Source: CAD feature listing. Evaluate the final solid. Frame: model axes, mm. A direction names the side the tool comes from. Coordinates: 2 decimals unless noted, no trailing zeros. Answer as a JSON object with one key per item and string values. Group by question number.
from build123d import *

# Parameters (mm, degrees)
F1_DEPTH = 7.874
F2_R     = 1.533026
F3_R     = 1.594347
F4_R     = 0.61321


with BuildPart() as f1:
    # F0 (on Front) → F1 (new body)
    with BuildSketch(Plane.XZ):
        Polygon((-7.47635, 9.42706), (-7.47635, 4.603866), (-8.243676, 4.603866), (-8.243676, 9.372251), (-24.138292, 9.372251), (-24.138292, 0), (0, 0), (0, 9.42706), align=None)
    extrude(amount=F1_DEPTH)

    # F2
    f2_edges = [f1.edges().sort_by_distance(p)[0] for p in [
        (-8.243676, -3.937, 9.372251),
    ]]
    fillet(f2_edges, radius=F2_R)

    # F3
    f3_edges = [f1.edges().sort_by_distance(p)[0] for p in [
        (-24.138292, -3.937, 9.372251),
        (-7.47635, -3.937, 9.42706),
    ]]
    fillet(f3_edges, radius=F3_R)

    # F4
    f4_edges = [f1.edges().sort_by_distance(p)[0] for p in [
        (-8.243676, -3.937, 4.603866),
    ]]
    fillet(f4_edges, radius=F4_R)

    # F5: F1 across face


with BuildPart() as f1_1:
    add(f1.part)
    add(f1.part.mirror(Plane(origin=(0, -3.937, 4.71353), x_dir=(0, 1, 0), z_dir=(1, 0, 0))))

    # F6: F1 across face


with BuildPart() as f1_2:
    add(f1_1.part)
    add(f1_1.part.mirror(Plane(origin=(0, -3.937, 0), x_dir=(1, 0, 0), z_dir=(0, 0, -1))))


solid = f1_2.part
1. Ray query, L1, parallel to X at y = -6.25, z = 6.5; L2, parallel to X at y = -3, z = -8; L3, parallel to Z at x = 20.5, y = -0.25. Return the intervals inside material, ascending.
2. Reachability of faces 1 (the face through (16, -4, -9.372)), 2 (the face through (-16, -4, 9.372)), 3 (the face through (8.244, -4, 7)), 4 (the face through (7.02, -3.99, -8.95)) from +Z, -Z, +X, -X, +Y, -Y: full face, straight path, thin tool, end or side. Return the list, or none.
3. Mould query, pull axis X, two halves, no side actions, for faces 5 (the face through (8.68, -3.99, -8.91)), 6 (the face through (16, -4, 9.372)), 7 (the face through (-23.659, -3.992, 8.918)), 8 (the face through (-8.244, -4, 7)). Classes: pulls with the +X half, pulls with the -X half, needs draft (parallel to the pull), parting line crosses it, or undercut.
4. Pin query (flat end, axial travel): pin 1 Ø2 at (x, y) = (12, -4) entering from +Z; pin 2 Ø2.5 at (x, y) = (-15.5, -5.5) entering from -Z. Return the tip coordinate at first contact, or that it passes through.
Solved:
{
 "1": {"L1": "-24.14 to -8.24, -7.48 to 7.48, 8.24 to 24.14", "L2": "-24.12 to -8.25, -7.47 to 7.47, 8.25 to 24.12", "L3": "-9.37 to 9.37"},
 "2": {"face 1": "-Z, +X, +Y, -Y", "face 2": "+Z, -X, +Y, -Y", "face 3": "+Z, +Y, -Y", "face 4": "-Z, +Y, -Y"},
 "3": {"face 5": "undercut", "face 6": "needs draft", "face 7": "pulls with the -X half", "face 8": "undercut"},
 "4": {"pin 1": "z = 9.37", "pin 2": "z = -9.37"}
}
